Model file for the job. Use its own axes, mm. Give positions to 0.01 mm unless a question says otherwise; leave off trailing zeros. Order: outer loops, then holes, each group sorted by start corner. A loop starts at its lowest first (then second) coordinate and runs counter-clockwise, first axis right, second up. Notation, with made-up numbers: (57.5, 15) -> (88.5, 15) arc R20 ccw to (88.5, 30) -> close; hole circle Ø7 at (79, -34). An arc over 180 degrees is marked (long way). Use CSV: the item, a comma, the result in double quotes. Start each with the question number.
1. Cut at B-B on z = -54.5. List the corners of the cut face in (x, y) (3 decimals), then the cut area to 3 significant figures.
2. Cut at A-A on x = 4.5. List the corners of the cut face in (y, z) (3 decimals), then the cut area to 3 significant figures.
3. Wall check: line 1 (X direction, y = 1.75, z = -26.5) (3 decimals); line 2 (Z direction, x = 87.5, y = 0.5) (3 decimals); line 3 (Z direction, x = -52, y = 4.5) (3 decimals). Give the ranges that are in metal, low to high. Write a range as from..to.
4. Pull direction Z, two halves, no side cores. Call faces 1 (the flat face through (-1, 3, -85.09)), 2 (the flat face through (-1, 3, 85.09)), 3 (the flat face through (16, 3.175, 0)), 4 (the flat face through (15, 0, 6)): released by +Z, released by -Z, zero draft, split by the parting line, or undercut.
5. Drop flat-ended pins along their axis: pin 1 (3 mm diameter, centred on x = -98.425, z = -60.452, fed in from -Y); pin 2 (5.5 mm diameter, centred on x = 15.875, z = -60.452, fed in from -Y); pin 3 (4 mm diameter, centred on x = -98.425, z = 60.452, fed in from +Y) (3 decimals). Give the stop position or say it passes through.
6. Cut at C-C on y = 1.75. List the corners of the cut face in (x, z) (3 decimals), then the cut area to 3 significant figures.
```python
from build123d import *

# Parameters (mm, degrees)
SKETCH1_W                 = 203.2
SKETCH1_H                 = 170.18
BOSS_EXTRUDE1_DEPTH       = 6.35
SKETCH3_W                 = 151.13
SKETCH3_H                 = 3.175
CUT_EXTRUDE1_DEPTH        = 204.2
SKETCH4_W                 = 104.775
SKETCH4_H                 = 138.43
SKETCH4_W_2               = 73.025
CUT_EXTRUDE3_DEPTH        = 4.175
M4X0_7_TAPPED_HOLE1_D     = 3.3
M4X0_7_TAPPED_HOLE1_DEPTH = 9.906


with BuildPart() as part:
    # Sketch1 → Boss-Extrude1 (new body)
    with BuildSketch(Plane(origin=(0, 0, 0), x_dir=(1, 0, 0), z_dir=(0, 1, 0))):
        Rectangle(SKETCH1_W, SKETCH1_H)
    extrude(amount=BOSS_EXTRUDE1_DEPTH)

    # Sketch3 → Cut-Extrude1 (cut, through all)
    with BuildSketch(Plane(origin=(101.6, 0, 0), x_dir=(0, 0, -1), z_dir=(1, 0, 0))):
        with Locations((0, 4.7625)):
            Rectangle(SKETCH3_W, SKETCH3_H)
    extrude(amount=-CUT_EXTRUDE1_DEPTH, mode=Mode.SUBTRACT)

    # Sketch4 → Cut-Extrude3 (cut, through all)
    with BuildSketch(Plane(origin=(0, 3.175, 0), x_dir=(1, 0, 0), z_dir=(0, 1, 0))):
        with Locations((-42.8625, 0)):
            Rectangle(SKETCH4_W, SKETCH4_H)
        with Locations((58.7375, 0)):
            Rectangle(SKETCH4_W_2, SKETCH4_H)
    extrude(amount=-CUT_EXTRUDE3_DEPTH, mode=Mode.SUBTRACT)

    # M4x0.7 Tapped Hole1
    with Locations(Plane(origin=(0, 3.175, 0), x_dir=(1, 0, 0), z_dir=(0, 1, 0))):
        with Locations((-98.425, -60.452), (-98.425, 60.452), (15.875, 60.452), (15.875, -60.452)):
            Hole(M4X0_7_TAPPED_HOLE1_D / 2, depth=M4X0_7_TAPPED_HOLE1_DEPTH)


solid = part.part
```
Verdict:
1,outline,"(-101.6, 0) -> (-95.25, 0) -> (-95.25, 3.175) -> (-101.6, 3.175) -> close; (9.525, 0) -> (22.225, 0) -> (22.225, 3.175) -> (9.525, 3.175) -> close; (95.25, 0) -> (101.6, 0) -> (101.6, 3.175) -> (95.25, 3.175) -> close"
1,area,"80.6 mm^2"
2,outline,"(0, -85.09) -> (6.35, -85.09) -> (6.35, -75.565) -> (3.175, -75.565) -> (3.175, -69.215) -> (0, -69.215) -> close; (0, 69.215) -> (3.175, 69.215) -> (3.175, 75.565) -> (6.35, 75.565) -> (6.35, 85.09) -> (0, 85.09) -> close"
2,area,"161 mm^2"
3,line 1,"-101.6..-95.25, 9.525..22.225, 95.25..101.6"
3,line 2,"-85.09..-69.215, 69.215..85.09"
3,line 3,"-85.09..-75.565, 75.565..85.09"
4,face 1,"released by -Z"
4,face 2,"released by +Z"
4,face 3,"undercut"
4,face 4,"zero draft"
5,pin 1,"through"
5,pin 2,"y = 0"
5,pin 3,"y = 3.175"
6,outline,"(-101.6, -85.09) -> (101.6, -85.09) -> (101.6, 85.09) -> (-101.6, 85.09) -> close; hole circle Ø3.3 at (-98.425, -60.452); hole circle Ø3.3 at (-98.425, 60.452); hole (-95.25, -69.215) -> (9.525, -69.215) -> (9.525, 69.215) -> (-95.25, 69.215) -> close; hole circle Ø3.3 at (15.875, -60.452); hole circle Ø3.3 at (15.875, 60.452); hole (22.225, -69.215) -> (95.25, -69.215) -> (95.25, 69.215) -> (22.225, 69.215) -> close"
6,area,"9,930 mm^2"
